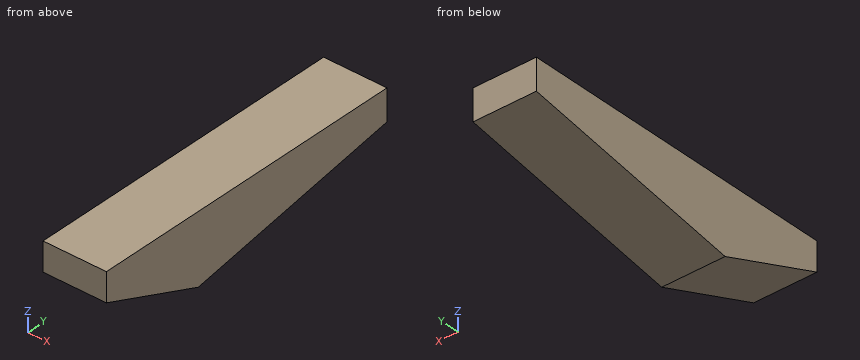
Autodesk Inventor part; units mm, degrees
ref_plane "XZ Plane" through (0, 0, 0) normal (0, 1, 0) x (-1, 0, 0)
sketch "BoundingBox" plane through (0, 0, 0) normal (1, 0, 0) x (0, 1, 0)
  line L0 (434.8115, 24.0504) -> (-18, 24.0504)
  line L1 (-18, 24.0504) -> (-18, -15.6719)
  line L2 (-18, -15.6719) -> (130.2861, -72.3729)
  line L3 (130.2861, -72.3729) -> (434.8115, -19.2646)
  line L4 (434.8115, -19.2646) -> (434.8115, 24.0504)
  point P0 (0, 0)
  point P1 (417.3115, 0.6447)
  point P2 (-18, 4.1892)
  dimension "d5" = 24.0504
  dimension "d6" = 4.1893
  dimension "d7" = 110.926
  dimension "d8" = 452.8115
  dimension "d9" = 39.7223
  dimension "d10" = 43.315
  dimension "d11" = 99.893
  dimension "d12" = 56.7009
  dimension "d13" = 17.5
  dimension "d14" = 23.4057
extrude "BoundingBoxFeature" add sketch "BoundingBox" along normal mid plane 88
properties part number "UpperArmBoundingBox"
Verification items for the finished model (mm, model axes). Give positions to 0.01 mm unless a question says otherwise; leave off trailing zeros. Write each loop counter-clockwise with the first axis right and the second up, starting at its lowest first coordinate (ties: lowest second). Pieces come first, ordered by that corner, then holes. Notation, with made-up numbers: M 71.25,10 L 126.25,10 A25 cw 126.25,23 Z; hole C -39,34.5 d9. An arc over 180 degrees is marked long. Write item = value, one per line.
(1) Material ranges on line 1 (Z direction, x = -25.5, y = 355); line 2 (Z direction, x = -24.5, y = 258), recorded low to high.
Found:
line_1 = -33.18 to 24.05
line_2 = -50.1 to 24.05
(2) Sectioned sample at C-C (z = -53). Record the cut outline in (x, y).
Found:
outline = M -44,79.62 L 44,79.62 L 44,241.37 L -44,241.37 Z
(3) Sectioned sample at B-B (y = 270). Record the cut outline in (x, z), then the cut area to 3 significant figures.
Found:
outline = M -44,-48.01 L 44,-48.01 L 44,24.05 L -44,24.05 Z
area = 6,340 mm2
(4) Go/stop test with flat-tipped pins: pin 1 Ø5 at (x, y) = (1.5, 77) entering from -Z; pin 2 Ø5 at (x, y) = (-8, 387) entering from -Z. Record where each tip stops, or that it passes through.
Found:
pin_1 = -52.95
pin_2 = -28.04
(5) Sectioned sample at A-A (x = 29). Record the cut outline in (y, z), then the cut area to 3 significant figures.
Found:
outline = M -18,-15.67 L 130.29,-72.37 L 434.81,-19.26 L 434.81,24.05 L -18,24.05 Z
area = 31,400 mm2
